The drawing under review shows one solid part. Ordinate dimensions are in mm from its lowest x, y, z. Give positions to 0.01 mm unless a question says otherwise; leave off trailing zeros. Write each loop counter-clockwise with the first axis right and the second up, starting at its lowest first coordinate (ties: lowest second). Pieces come first, ordered by that corner, then holes. Notation, with made-up numbers: (25.5, -27) -> (69.5, -27) arc R25 ccw to (69.5, -12) -> close; hole circle Ø5 at (-29.5, 6.25). An arc over 180 degrees is marked (long way). Put each result on its own line as item: value. Start each with the question number.
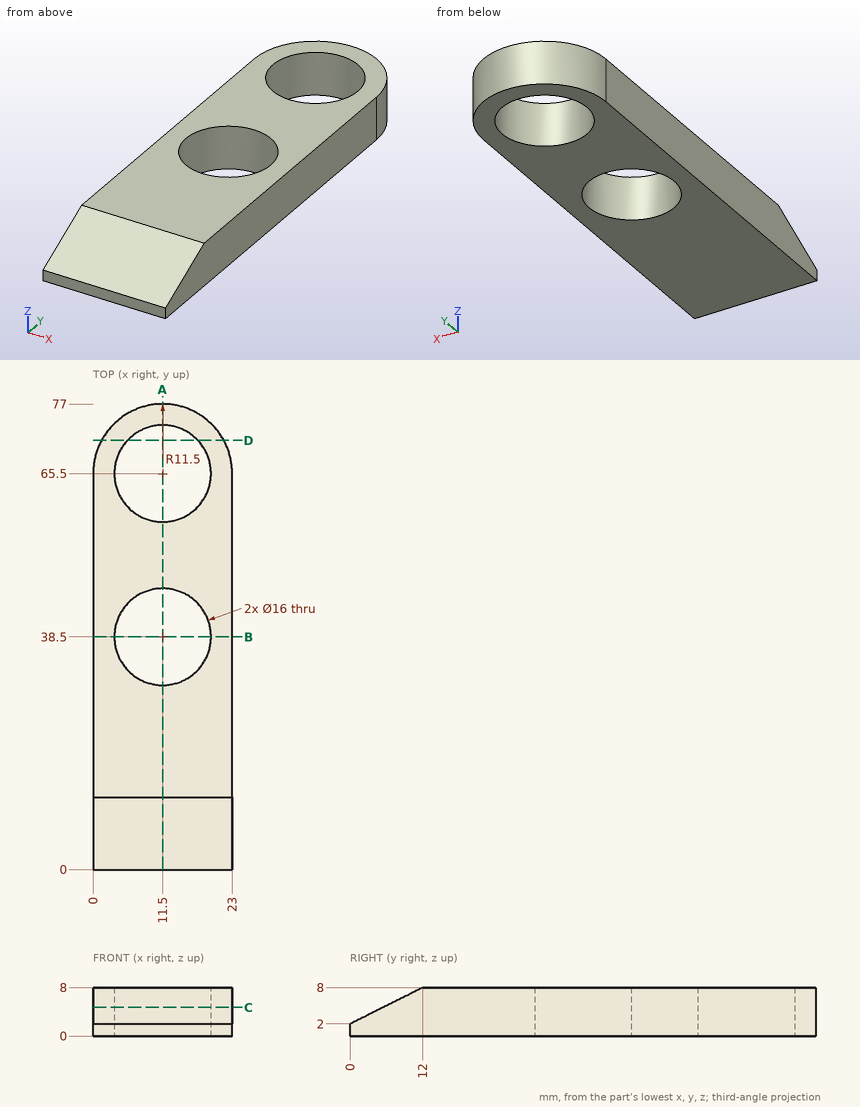
Q1. Take a section at C-C on z = 4.75. Give the boundary of the cut face in (x, y), then the cut area to 3 significant figures.
Q2. Take a section at B-B on y = 38.5. Give the boundary of the cut face in (x, z), then the cut area to 3 significant figures.
Q3. To check wall thickness, follow probe 1 along Y at (x, z) = (11, 1.5); probe 2 along Y at (x, z) = (7, 7); probe 3 along X at (y, z) = (66.5, 1). State the ranges of each line that lie inside material, in increasing order. Write a range as from..to.
Q4. Take a section at D-D on y = 71. Give the boundary of the cut face in (x, z).
Q5. For pin 1 (13 mm diameter, centred on x = 11.5, y = 65.5, fed in from +Z), flat-tipped, find the tip position at first contact; note if it passes through.
Q6. Take a section at A-A on x = 11.5. Give the boundary of the cut face in (y, z), then the cut area to 3 significant figures.
Result:
1. outline: (0, 5.5) -> (23, 5.5) -> (23, 65.5) arc R11.5 ccw to (0, 65.5) -> close; hole circle Ø16 at (11.5, 38.5); hole circle Ø16 at (11.5, 65.5)
1. area: 1,190 mm^2
2. outline: (0, 0) -> (3.5, 0) -> (3.5, 8) -> (0, 8) -> close; (19.5, 0) -> (23, 0) -> (23, 8) -> (19.5, 8) -> close
2. area: 56.0 mm^2
3. probe 1: y = 0..30.52, 46.48..57.52, 73.48..76.99
3. probe 2: y = 10..31.89, 45.11..58.89, 72.11..76.08
3. probe 3: x = 0.04..3.56, 19.44..22.96
4. outline: (1.4, 0) -> (5.69, 0) -> (5.69, 8) -> (1.4, 8) -> close; (17.31, 0) -> (21.6, 0) -> (21.6, 8) -> (17.31, 8) -> close
5. pin 1: passes through
6. outline: (0, 0) -> (30.5, 0) -> (30.5, 8) -> (12, 8) -> (0, 2) -> close; (46.5, 0) -> (57.5, 0) -> (57.5, 8) -> (46.5, 8) -> close; (73.5, 0) -> (77, 0) -> (77, 8) -> (73.5, 8) -> close
6. area: 324 mm^2
